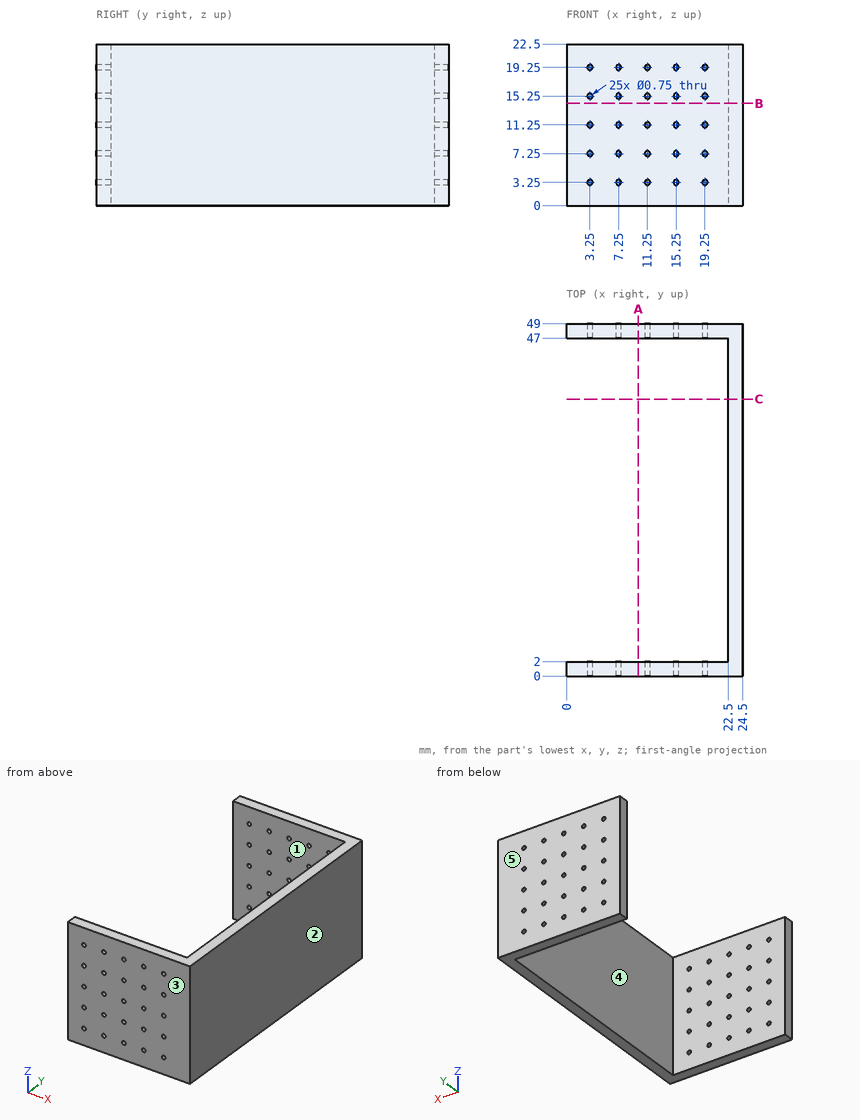
Job drawing, mm, ordinate dimensions from the low corner. One solid piece. A direction names the side the tool comes from. Give positions to 0.01 mm unless a question says otherwise; leave off trailing zeros. Order: outer loops, then holes, each group sorted by start corner. A loop starts at its lowest first (then second) coordinate and runs counter-clockwise, first axis right, second up. Notation, with made-up numbers: (85.5, -12.75) - (132.5, -12.75) arc R17 ccw to (132.5, 1.25) - close; hole circle Ø1 at (53.25, -5.5). An arc over 180 degrees is marked (long way). Return JSON: item names as keys, results as strings.
1) Cut at B-B, the plane z = 14.25. Give the cut face in (x, y), plus the area to 3 significant figures.
Geometry says:
{"outline": "(0, 0) - (24.5, 0) - (24.5, 49) - (0, 49) - (0, 47) - (22.5, 47) - (22.5, 2) - (0, 2) - close", "area": "188 mm²"}
2) 3-axis set-ups, long thin cutter, end or side, ignore diameter. For the marked faces 4 and 5: which of +Z, -Z, +X, -X, +Y, -Y reach the whole face in a straight line?
Geometry says:
{"face 4": "+Z, -Z, -X", "face 5": "+Z, -Z, +X, -X, +Y"}
3) Cut at A-A, the plane x = 10. Give the cut face in (y, z).
Geometry says:
{"outline": "(0, 0) - (2, 0) - (2, 22.5) - (0, 22.5) - close; (47, 0) - (49, 0) - (49, 22.5) - (47, 22.5) - close"}
4) Pull direction Y, two halves, no side cores. Call the marked faces 1, 2 and 3: pulls with the +Y half, pulls with the -Y half, needs draft (parallel to the pull), parting line crosses it, or undercut.
Geometry says:
{"face 1": "undercut", "face 2": "needs draft", "face 3": "pulls with the -Y half"}
5) Cut at C-C, the plane y = 38.5. Give the cut face in (x, z).
Geometry says:
{"outline": "(22.5, 0) - (24.5, 0) - (24.5, 22.5) - (22.5, 22.5) - close"}
6) Flat gauge pin, fed straight in: P1, Ø8, axis at y = 41, z = 8.5, coming from the -X side. Where does the tip first touch, or does it go through?
Geometry says:
{"P1": "x = 22.5"}
7) Probe line 1 (X direction, y = 48.4, z = 19.25) (3 decimals); line 2 (Z direction, x = 11.25, y = 1.15) (3 decimals); line 3 (Y direction, x = 16, z = 9.5). List the from-to ranges inside material, lowest first. Write a range as from..to.
Geometry says:
{"line 1": "0..2.875, 3.625..6.875, 7.625..10.875, 11.625..14.875, 15.625..18.875, 19.625..24.5", "line 2": "0..2.875, 3.625..6.875, 7.625..10.875, 11.625..14.875, 15.625..18.875, 19.625..22.5", "line 3": "0..2, 47..49"}
